The listing builds one solid part. Answer for the finished solid, in the listing's coordinates (mm). A direction names the side the tool comes from. Coordinates: 2 decimals unless noted, no trailing zeros. Order: outer loops, then holes, each group sorted by start corner. A loop starts at its lowest first (then second) coordinate and runs counter-clockwise, first axis right, second up. Notation, with made-up numbers: (79.5, -1.75) -> (117.5, -1.75) arc R23 cw to (117.5, 16.25) -> close; hole circle Ø7 at (-17, -7). An arc over 180 degrees is marked (long way). Return JSON: item names as keys, results as strings.
Autodesk Inventor part; units mm, degrees
ref_plane "YZ Plane" through (0, 0, 0) normal (1, 0, 0) x (0, 1, 0)
ref_plane "XZ Plane" through (0, 0, 0) normal (0, 1, 0) x (-1, 0, 0)
ref_plane "XY Plane" through (0, 0, 0) normal (0, 0, 1) x (1, 0, 0)
sketch "Boceto1" plane through (0, 0, 0) normal (0, 0, 1) x (1, 0, 0)
  circle A0 centre (0, 0) radius 7
  dimension "d0" = 14
extrude "Extrusión1" add sketch "Boceto1" along normal blind 20
sketch "Boceto2" plane through (0, 0, 0) normal (0, 0, -1) x (-1, 0, 0)
  circle A0 centre (0, 0) radius 1
  dimension "d3" = 2
extrude "Extrusión2" cut sketch "Boceto2" against normal blind 2.5
sketch "Boceto3" plane through (0, 0, 20) normal (0, 0, 1) x (1, 0, 0)
  circle A0 centre (0, 0) radius 3
  dimension "d6" = 6
extrude "Extrusión3" add sketch "Boceto3" along normal blind 20
properties part number "pendulum_coupling"
1. For faces 4 (the face through (0, 0, 40)), 5 (the face through (1, -3, 20)), 6 (the face through (0, -1, 1)), determine the directions among +Z, -Z, +X, -X, +Y, -Y from which every point of the face is accessible in a straight line to the end or side of a thin tool.
Answer block:
{"face 4": "+Z, +X, -X, +Y, -Y", "face 5": "+Z", "face 6": "-Z"}
2. Determine the mould class of faces 1 (the face through (6.466, 2.681, 9.86)), 2 (the face through (-0.1, -1.5, 0)), 3 (the face through (0, 0, 2.5)) for opening direction X: pulls with the +X half, pulls with the -X half, needs draft (parallel to the pull), parting line crosses it, or undercut.
Answer block:
{"face 1": "parting line crosses it", "face 2": "needs draft", "face 3": "undercut"}
3. The part is cut by section A-A on x = 0. Give the vertices of the cut face in (y, z).
Answer block:
{"outline": "(-7, 0) -> (-1, 0) -> (-1, 2.5) -> (1, 2.5) -> (1, 0) -> (7, 0) -> (7, 20) -> (3, 20) -> (3, 40) -> (-3, 40) -> (-3, 20) -> (-7, 20) -> close"}
4. Each of these flat-tipped pins is pushed along its axis until it touches: pin 1 Ø1 at (x, z) = (-5, 22.5) entering from -Y; pin 2 Ø2 at (x, z) = (2.5, 8) entering from +Y; pin 3 Ø5 at (x, z) = (4.5, 23) entering from +Y; pin 4 Ø5 at (y, z) = (-5, 9.5) entering from +X. Where does it stop, or does it pass through?
Answer block:
{"pin 1": "passes through", "pin 2": "stops at y = 6.84", "pin 3": "stops at y = 2.24", "pin 4": "stops at x = 6.54"}
5. Consider line 1 (Y direction, x = 0, z = 1.05); line 2 (Z direction, x = -5.25, y = 2); line 3 (Y direction, x = 3, z = 9). Determine where each line is inside the solid, lowest interval first. Write a range as from..to.
Answer block:
{"line 1": "y = -7..-1, 1..7", "line 2": "z = 0..20", "line 3": "y = -6.32..6.32"}
6. The part is cut by section D-D on y = 1.75. Give the vertices of the cut face in (x, z), and give its area (3 significant figures).
Answer block:
{"outline": "(-6.78, 0) -> (6.78, 0) -> (6.78, 20) -> (2.44, 20) -> (2.44, 40) -> (-2.44, 40) -> (-2.44, 20) -> (-6.78, 20) -> close", "area": "369 mm2"}
7. The part is cut by section C-C on z = 15. Give the vertices of the cut face in (x, y).
Answer block:
{"outline": "circle Ø14 at (0, 0)"}
